Geometry: final body of the model. Coordinates: model frame, mm. A direction names the side the tool comes from. Coordinates: 2 decimals unless noted, no trailing zeros. Loops run counter-clockwise (first coordinate to the right, second up) from the corner with the lowest first, then second, coordinate; pieces in that order, holes last. Notation, with made-up numbers: (74, 68.25) - (96, 68.25) arc R16 cw to (96, 95.25) - close; hole circle Ø10 at (-24.5, -37.75). An arc over 180 degrees is marked (long way). Put each result on its own line as item: value. Start each with the question number.
1) Section A-A on z = 0. Output: boundary loops of the cut face in (x, y).
2) Draft query along Y for faces 1 (the cylindrical face through (-1.479, -5.158, -3.955)), 2 (the flat face through (7, 0, -3)), 3 (the cylindrical face through (2.81, -0.596, -2.685)). Return one class per face: +Y half, -Y half, draft (parallel to the pull), parting line (faces both ways), or undercut.
3) Reachability of faces 4 (the flat face through (0, 0, -6)), 5 (the flat face through (-3, 1.4, -4.2)), 6 (the cylindrical face through (0.74, 2.58, -4.05)) from +Z, -Z, +X, -X, +Y, -Y: full face, straight path, thin tool, end or side. Return the list, or none.
4) Section C-C on x = -1. Output: boundary loops of the cut face in (y, z), and give its area (3 significant figures).
5) Contact query for flat-ended pins moving along their axis: pin 1 Ø5 at (y, z) = (0, 0) entering from +X; pin 2 Ø2 at (x, z) = (5, -1) entering from +Y; pin 3 Ø1 at (x, y) = (3, -5) entering from -Z; pin 4 Ø5 at (x, y) = (4.5, -2.5) entering from +Z. Output: stop coordinate, or through.
6) Section B-B on x = 0.75. Output: boundary loops of the cut face in (y, z).
7) Material intervals for line 1 along Z through (x, y) = (2, 0); line 2 along X through (y, z) = (0.25, 6); line 3 along Y through (x, z) = (-1, -2.5), sorted ascending. Write a range as from..to.
Autodesk Inventor part; units mm, degrees
ref_plane "YZ Plane" through (0, 0, 0) normal (1, 0, 0) x (0, 1, 0)
ref_plane "XZ Plane" through (0, 0, 0) normal (0, 1, 0) x (-1, 0, 0)
ref_plane "XY Plane" through (0, 0, 0) normal (0, 0, 1) x (1, 0, 0)
sketch "Skizze1" plane through (0, 0, 0) normal (0, 0, 1) x (1, 0, 0)
  line L0 (-2.5, 0) -> (5.5, 0)
  line L1 (7, 2.75) -> (7, 5)
  line L2 (7, 5) -> (2, 5)
  line L3 (-3, 2.75) -> (-3, 6.5)
  line L4 (-3, 6.5) -> (0, 6.5)
  line L5 (2, 5) -> (1.3045, 4.8136)
  line L6 (1.2009, 4.8) -> (0.3, 4.8)
  line L7 (-0.0913, 5.2832) -> (0, 5.7125)
  line L8 (0, 5.7125) -> (0, 6.5)
  arc A0 (-0.0913, 5.2832) -> (0.3, 4.8) centre (0.3, 5.2) ccw
  arc A1 (1.2009, 4.8) -> (1.3045, 4.8136) centre (1.2009, 5.2) ccw
  line L9 (-28.4, 0) -> (128.4, 0)
  line L10 (0, -12) -> (0, 72)
  line L11 (-3, 2.75) -> (7, 2.75)
  dimension "d0" = 13
  dimension "d1" = 10
  dimension "d2" = 10
  dimension "d3" = 12
  dimension "d4" = 0.4
  dimension "d5" = 0.1
  dimension "d6" = 2
  dimension "d7" = 15
  dimension "d8" = 0.2
  dimension "d9" = 0.4
  dimension "d10" = 3
  dimension "d11" = 5.5
revolve "Körper" add sketch "Skizze1" angle 360 about axis through (-2.5, 0, 0) along (1, 0, 0) contours L11 L10 A0 L6 A1 L5 L2 L1 | L11 L3 L4 L8 L7 A0 L10
chamfer "Fase1" distance 1.25 angle 15 1 edges at (7, -5, 0) measured on face at (5.3333, 4.9353, -0.8021)
fillet "Rundung1" radius 1.5 1 edges at (-3, -2.75, 0)
equation "\"d12\" = PHH"
equation "\"d13\" = ANG"
equation "\"d29\" = PHH"
equation "\"d14\" = RR"
equation "\"d0\" = KOD"
equation "\"d1\" = SD2"
equation "\"d2\" = NLG"
equation "\"d4\" = FSRR"
equation "\"d5\" = FST2"
equation "\"d6\" = FSB"
equation "\"d8\" = FST1"
equation "\"d9\" = FSRR"
equation "\"d10\" = KOH"
equation "\"d11\" = NND"
equation "\"NLG\" = 10"
equation "\"NND\" = 5.5"
equation "\"KOD\" = 13"
equation "\"KOH\" = 3"
equation "\"SD2\" = 10"
equation "\"FST1\" = 0.2"
equation "\"FST2\" = 0.1"
equation "\"FSB\" = 2"
equation "\"FSRR\" = 0.4"
equation "\"PHH\" = 1.25"
equation "\"ANG\" = 15deg"
equation "\"RR\" = 1.5"
equation "\"NNDMIN\" = 5.1"
equation "\"FSH\" = 1.1"
equation "\"NNDMAX\" = 6"
equation "\"SEWI\" = 30deg"
properties part number "DIN 172 - A 5,5 x 10" material "Stahl, weich"
Answer block:
1. outline: (-3, -6.5) - (0, -6.5) - (0, -5.71) - (-0.09, -5.28) arc R0.4 cw to (0.3, -4.8) - (1.2, -4.8) arc R0.4 cw to (1.3, -4.81) - (2, -5) - (5.75, -5) - (7, -4.67) - (7, -2.75) - (-1.5, -2.75) arc R1.5 ccw to (-3, -4.25) - close; (-3, 4.25) arc R1.5 ccw to (-1.5, 2.75) - (7, 2.75) - (7, 4.67) - (5.75, 5) - (2, 5) - (1.3, 4.81) arc R0.4 cw to (1.2, 4.8) - (0.3, 4.8) arc R0.4 cw to (-0.09, 5.28) - (0, 5.71) - (0, 6.5) - (-3, 6.5) - close
2. face 1: parting line
2. face 2: draft
2. face 3: undercut
3. face 4: +X
3. face 5: +Z, -Z, -X, +Y, -Y
3. face 6: none
4. outline: circle Ø13 at (0, 0); hole circle Ø5.5 at (0, 0)
4. area: 109 mm²
5. pin 1: passes through
5. pin 2: stops at y = 5
5. pin 3: stops at z = -2.18
5. pin 4: stops at z = 5
6. outline: circle Ø9.6 at (0, 0); hole circle Ø5.5 at (0, 0)
7. line 1: z = -5..-2.75, 2.75..5
7. line 2: x = -3..0
7. line 3: y = -6..-1.15, 1.15..6
